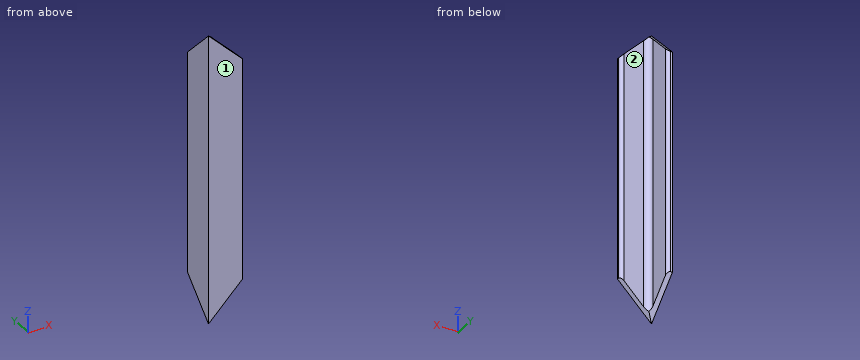
Autodesk Inventor part; units mm, degrees
ref_plane "Start plane" through (0, 0, -10) normal (0, 0, 1) x (1, 0, 0)
ref_plane "End plane" through (0, 0, 160) normal (0, 0, 1) x (1, 0, 0)
ref_plane "Work Plane11" through (-6, 4, 160) normal (0.7071, 0, 0.7071) x (0.7071, 0, -0.7071)
ref_plane "Start plane" through (0, 0, -10) normal (0, 0, 1) x (1, 0, 0)
ref_plane "End plane" through (0, 0, 160) normal (0, 0, 1) x (1, 0, 0)
sketch "Sketch" plane through (0, 0, 0) normal (0, 0, 1) x (1, 0, 0)
  line L0 (-3, 0.5) -> (-3, 12)
  line L1 (-6, 14) -> (-5, 14)
  line L2 (-6, -6) -> (-6, 14)
  line L3 (-6, -6) -> (14, -6)
  line L4 (14, -5) -> (14, -6)
  line L5 (0.5, -3) -> (12, -3)
  arc A0 (-3, 0.5) -> (0.5, -3) centre (0.5, 0.5) ccw
  arc A1 (-3, 12) -> (-5, 14) centre (-5, 12) ccw
  arc A2 (14, -5) -> (12, -3) centre (12, -5) ccw
  line L6 (0, 18.4971) -> (0, -10.0828) construction
  line L7 (-10.0828, 0) -> (18.4971, 0) construction
  point P0 (-3, -3)
  point P1 (-3, 14)
  point P2 (14, -3)
  dimension "d4" = 20
  dimension "d6" = 20
  dimension "d8" = 3
  dimension "d10" = 3
  dimension "d17" = 3.5
  dimension "d18" = 2
  dimension "d19" = 6
  dimension "d20" = 6
extrude "Body" add sketch "Sketch" along normal up to surface (170 mm away) from surface at -10
sketch "Sketch3" plane through (0, 0, 0) normal (0, 0, 1) x (1, 0, 0)
  line L0 (0, 0) -> (10, 0)
ref_plane "Work Plane10" through (0, 0, 0) normal (0, -1, 0) x (1, 0, 0)
sketch "Sketch4" plane through (0, 0, 0) normal (0, -1, 0) x (1, 0, 0)
  line L0 (-2, -10) -> (12, -10)
  line L1 (-2, 160) -> (12, 160)
  dimension "d24" = 170
ref_plane "Work Plane11" through (-6, 4, 160) normal (0.7071, 0, 0.7071) x (0.7071, 0, -0.7071)
split "Split1" plane through (-6, 4, 160) removes the side toward (0.7071, 0, 0.7071)
ref_plane "Work Plane12" through (-6, 4, -10) normal (0.7071, 0, -0.7071) x (-0.7071, 0, -0.7071)
split "Split2" plane through (-6, 4, -10) removes the side toward (0.7071, 0, -0.7071)
ref_plane "Work Plane13" through (4, -6, -10) normal (0, 0.7071, -0.7071) x (1, 0, 0)
split "Split3" plane through (4, -6, -10) removes the side toward (0, 0.7071, -0.7071)
ref_plane "Work Plane14" through (4, -6, 160) normal (0, 0.7071, 0.7071) x (1, 0, 0)
split "Split4" plane through (4, -6, 160) removes the side toward (0, 0.7071, 0.7071)
equation "\"d4\" = b"
equation "\"d6\" = b"
equation "\"d17\" = R"
equation "\"d18\" = R1"
equation "\"d19\" = ex"
equation "\"d20\" = d19"
equation "\"d11\" = G_L"
equation "\"b\" = 20"
equation "\"ParT\" = 3"
equation "\"R\" = 3.5"
equation "\"R1\" = 2"
equation "\"G_L\" = d24"
equation "\"ex\" = 6"
equation "\"G_OFFSET_START\" = 10"
equation "\"G_OFFSET_END\" = 10"
equation "\"d21\" = -G_OFFSET_START"
equation "\"d22\" = G_OFFSET_END + B_L"
equation "\"B_L\" = 150"
properties part number "ISO 657-1 - L20x20x3-170" material "Stainless Steel"
Source: CAD feature listing. Evaluate the final solid. Frame: model axes, mm. Face numbers are marked on the shaded views. A direction names the side the tool comes from. Give positions to 0.01 mm unless a question says otherwise; leave off trailing zeros. Order: outer loops, then holes, each group sorted by start corner. A loop starts at its lowest first (then second) coordinate and runs counter-clockwise, first axis right, second up. Notation, with made-up numbers: (11.5, 48.25) -> (23.5, 48.25) arc R21 cw to (23.5, 60.25) -> close; hole circle Ø4 at (50.5, -2.5). An arc over 180 degrees is marked (long way). Use a Markdown table: item, result.
Q1. First-contact query: P1, Ø3.5, axis at x = 4, z = 75.5, coming from the +Y side; P2, Ø8, axis at x = 5.5, y = -3.5, coming from the -Z side; P3, Ø1, axis at y = 4, z = 8.5, coming from the +X side. Flat tips, straight axial feed; report the tip coordinate or a pass-through.
A:
| item | result |
|---|---|
| P1 | y = -3 |
| P2 | z = -2.5 |
| P3 | x = -3 |
Q2. Section B-B (x = 7.25). Return the cut outline in (y, z), and give its area (4 significant figures).
A:
| item | result |
|---|---|
| outline | (-6, 3.25) -> (-3, 3.25) -> (-3, 146.75) -> (-6, 146.75) -> close |
| area | 430.5 mm^2 |
Q3. Access query for the marked faces 1 and 2. Directions: +Z, -Z, +X, -X, +Y, -Y. A direction counts if a zero-diameter tool reaches every point of the face in a straight line with its end or side. Return the directions, or none.
A:
| item | result |
|---|---|
| face 1 | +Z, -Z, +X, -X, -Y |
| face 2 | +Z, -Z, +X, +Y |
Q4. Section C-C (y = 8.5). Return the cut outline in (x, z).
A:
| item | result |
|---|---|
| outline | (-6, 4.5) -> (-3, 4.5) -> (-3, 145.5) -> (-6, 145.5) -> close |
Q5. Section A-A (z = 65.5). Return the cut outline in (x, y), and give its area (3 significant figures).
A:
| item | result |
|---|---|
| outline | (-6, -6) -> (14, -6) -> (14, -5) arc R2 ccw to (12, -3) -> (0.5, -3) arc R3.5 cw to (-3, 0.5) -> (-3, 12) arc R2 ccw to (-5, 14) -> (-6, 14) -> close |
| area | 112 mm^2 |
Q6. Material intervals for line 1 (Y direction, x = -2, z = 71.5); line 2 (X direction, y = 1, z = 132.5), sorted ascending. Write a range as [from, to].
A:
| item | result |
|---|---|
| line 1 | [-6, -1.95] |
| line 2 | [-6, -3] |
